Geometry check sheet. Reference: the model listing, model coordinates, mm. A direction names the side the tool comes from. Round coordinates to 2 decimals unless told otherwise and drop trailing zeros. Loops run counter-clockwise (first coordinate to the right, second up) from the corner with the lowest first, then second, coordinate; pieces in that order, holes last. Notation, with made-up numbers: M 18,-7 L 29,-7 A16 cw 29,7 Z; hole C 61,-12 d1. An arc over 180 degrees is marked long. Answer in a Markdown table with one row per item. Add a question column.
```python
from build123d import *

# Parameters (mm, degrees)
F0_W     = 17
F0_H     = 50
F0_R     = 2.6
F0_R_2   = 3
F1_DEPTH = 8
F2_R     = 4
F2_R_2   = 3
F3_DEPTH = 1
F4_R     = 1.25
F5_DEPTH = 8


with BuildPart() as f1:
    # F0 (on Top) → F1 (new body)
    with BuildSketch(Plane.XY):
        with Locations((8.5, 25)):
            Rectangle(F0_W, F0_H)
        with Locations((8.5, 5.2)):
            Circle(F0_R, mode=Mode.SUBTRACT)
        with Locations((8.5, 18)):
            Circle(F0_R_2, mode=Mode.SUBTRACT)
        with Locations((8.219655, 44)):
            Circle(F0_R, mode=Mode.SUBTRACT)
        with Locations((8.5, 32)):
            Circle(F0_R_2, mode=Mode.SUBTRACT)
    extrude(amount=F1_DEPTH)

    # F2 (on face) → F3 (cut)
    with BuildSketch(Plane.XY.offset(8)):
        with Locations((8.5, 32)):
            Circle(F2_R)
        with Locations((8.5, 32)):
            Circle(F2_R_2, mode=Mode.SUBTRACT)
        with Locations((8.5, 18)):
            Circle(F2_R)
        with Locations((8.5, 18)):
            Circle(F2_R_2, mode=Mode.SUBTRACT)
    extrude(amount=-F3_DEPTH, mode=Mode.SUBTRACT)

    # F4 (on face) → F5 (cut)
    with BuildSketch(Plane(origin=(0, 50, 0), x_dir=(-1, 0, 0), z_dir=(0, 1, 0))):
        with Locations((-14, 4)):
            Circle(F4_R)
        with Locations((-3, 4)):
            Circle(F4_R)
    extrude(amount=-F5_DEPTH, mode=Mode.SUBTRACT)


solid = f1.part
```
1) Cross-section at B-B, the plane y = 32. Record the boundary of the cut face in (x, z).
2) Thickness scan on L1, parallel to X at y = 46, z = 3.5; L2, parallel to Z at x = 14, y = 48; L3, parallel to Y at x = 8.5, z = 7.3. Record the ranges inside material, lowest first. Write a range as [from, to].
3) Set-up check for faces 5 (the cylindrical face through (14.27, 46.06, 2.78)), 6 (the cylindrical face through (7.979, 35.966, 7.507)), 7 (the flat face through (8, 25, 0)): record each of +Z, -Z, +X, -X, +Y, -Y from which the full face is reachable in a straight line by a thin tool's end or side.
4) Cross-section at C-C, the plane z = 2.25. Record the boundary of the cut face in (x, y).
5) Cross-section at A-A, the plane y = 44. Record the boundary of the cut face in (x, z), plus the area to 3 significant figures.
6) Draft check along X on faces 1 (the flat face through (10, 21, 7)), 2 (the flat face through (0, 25, 4)), 3 (the flat face through (3, 42, 4)), 4 (the flat face through (8, 25, 8)). Enter one of: +X half, -X half, draft (parallel to the pull), parting line (faces both ways), or undercut.
7) Cross-section at D-D, the plane x = 3. Record the boundary of the cut face in (y, z), plus the area to 3 significant figures.
8) Go/stop test with flat-tipped pins: pin 1 (1 mm diameter, centred on x = 11.5, y = 34.5, fed in from +Z); pin 2 (1.2 mm diameter, centred on x = 14, z = 4.5, fed in from +Y). Record where each tip stops, or that it passes through.
Worked answers:
| question | item | result |
|---|---|---|
| 1 | outline | M 0,0 L 5.5,0 L 5.5,7 L 4.5,7 L 4.5,8 L 0,8 Z; M 11.5,0 L 17,0 L 17,8 L 12.5,8 L 12.5,7 L 11.5,7 Z |
| 2 | L1 | x = [0, 1.85], [4.15, 6.56], [9.88, 12.85], [15.15, 17] |
| 2 | L2 | z = [0, 2.75], [5.25, 8] |
| 2 | L3 | y = [0, 2.6], [7.8, 14], [22, 28], [36, 41.42], [46.58, 50] |
| 3 | face 5 | +Y |
| 3 | face 6 | +Z |
| 3 | face 7 | -Z, +X, -X, +Y, -Y |
| 4 | outline | M 0,0 L 17,0 L 17,50 L 0,50 Z; hole C 8.5,18 d6; hole C 8.5,32 d6; hole C 8.22,44 d5.2; hole C 8.5,5.2 d5.2 |
| 5 | outline | M 0,0 L 5.62,0 L 5.62,8 L 0,8 Z; M 10.82,0 L 17,0 L 17,8 L 10.82,8 Z; hole C 3,4 d2.5; hole C 14,4 d2.5 |
| 5 | area | 84.6 mm2 |
| 6 | face 1 | undercut |
| 6 | face 2 | -X half |
| 6 | face 3 | undercut |
| 6 | face 4 | draft |
| 7 | outline | M 0,0 L 50,0 L 50,2.75 L 42,2.75 L 42,5.25 L 50,5.25 L 50,8 L 0,8 Z |
| 7 | area | 380 mm2 |
| 8 | pin 1 | stops at z = 8 |
| 8 | pin 2 | stops at y = 42 |
